Autodesk Inventor part; units mm, degrees
ref_plane "YZ Plane" through (0, 0, 0) normal (1, 0, 0) x (0, 1, 0)
ref_plane "XZ Plane" through (0, 0, 0) normal (0, 1, 0) x (-1, 0, 0)
ref_plane "XY Plane" through (0, 0, 0) normal (0, 0, 1) x (1, 0, 0)
sketch "Sketch1" plane through (0, 0, 0) normal (0, 0, 1) x (1, 0, 0)
  line L0 (0, 0) -> (-2.0828, 0)
  line L1 (-2.0828, 0) -> (-2.0828, 9.144)
  line L2 (-2.0828, 9.144) -> (0, 9.144)
  line L3 (0, 9.144) -> (0, 0)
  line L4 (-2.0828, 9.144) -> (-3.81, 11.176)
  line L5 (-3.81, 11.176) -> (-3.81, 11.684)
  line L6 (-3.81, 11.684) -> (0, 11.684)
  line L7 (0, 11.684) -> (0, 9.144)
  dimension "d0" = 4.1656
  dimension "d1" = 9.144
  dimension "d2" = 7.62
  dimension "d3" = 0.508
  dimension "d4" = 2.54
revolve "Revolution1" add sketch "Sketch1" angle 360 about axis through (0, 9.144, 0) along (0, -1, 0)
thread "Thread1"
sketch "Sketch2" plane through (0, 11.684, 0) normal (0, 1, 0) x (1, 0, 0)
  circle A0 centre (0, 0) radius 3.81
  line L0 (2.54, 0.635) -> (2.54, -0.635)
  line L1 (-2.54, -0.635) -> (-2.54, 0.635)
  line L2 (-0.635, 2.54) -> (0.635, 2.54)
  line L3 (0.635, -2.54) -> (-0.635, -2.54)
  line L4 (-0.635, -2.54) -> (-0.635, -1.397)
  line L5 (-0.635, 1.397) -> (-0.635, 2.54)
  line L6 (2.54, -0.635) -> (1.397, -0.635)
  line L7 (-1.397, -0.635) -> (-2.54, -0.635)
  line L8 (0.635, 2.54) -> (0.635, 1.397)
  line L9 (0.635, -1.397) -> (0.635, -2.54)
  line L10 (-2.54, 0.635) -> (-1.397, 0.635)
  line L11 (1.397, 0.635) -> (2.54, 0.635)
  line L12 (0, 2.54) -> (0, 0) construction
  line L13 (0, 0) -> (-2.54, 0) construction
  arc A1 (-0.635, -1.397) -> (-1.397, -0.635) centre (-1.397, -1.397) ccw
  arc A2 (1.397, -0.635) -> (0.635, -1.397) centre (1.397, -1.397) ccw
  arc A3 (0.635, 1.397) -> (1.397, 0.635) centre (1.397, 1.397) ccw
  arc A4 (-1.397, 0.635) -> (-0.635, 1.397) centre (-1.397, 1.397) ccw
  dimension "d8" = 1.27
  dimension "d9" = 5.08
  dimension "d10" = 0.762
extrude "Extrusion1" cut sketch "Sketch2" against normal blind 2.54 draft -14 contours L0 L6 A2 L9 L3 L4 A1 L7 L1 L10 A4 L5 L2 L8 A3 L11
chamfer "Chamfer1" distance 0.254 angle 45 1 edges at (2.0828, 0, 0)
properties material "Steel"
Geometry: final body of the model. Coordinates: model frame, mm. A direction names the side the tool comes from. Round coordinates to 2 decimals unless told otherwise and drop trailing zeros. Loops run counter-clockwise (first coordinate to the right, second up) from the corner with the lowest first, then second, coordinate; pieces in that order, holes last.
Item 1: Contact query for flat-ended pins moving along their axis: P1, Ø3, axis at x = 2.5, y = 6, coming from the -Z side; P2, Ø1.5, axis at y = 4, z = -1.5, coming from the +X side; P3, Ø3, axis at y = 6, z = -1, coming from the -X side. Output: stop coordinate, or through.
Checked values:
P1: stops at z = -1.83
P2: stops at x = 1.94
P3: stops at x = -2.08
Item 2: Section A-A, the plane y = 6.75. Output: boundary loops of the cut face in (x, z), plus the area to 3 significant figures.
Checked values:
outline: circle Ø4.17 at (0, 0)
area: 13.6 mm2
Item 3: Line query: L1, parallel to Z at x = 1, y = 8.5; L2, parallel to Z at x = 2, y = 10.5. Output: solid intervals per line, ascending.
Checked values:
L1: z = -1.83 to 1.83
L2: z = -2.54 to -0.34, 0.34 to 2.54
Item 4: Reachability of faces 1 (the flat face through (0, 0, 0)), 2 (the cylindrical face through (-1.987, 4.761, 0.626)), 3 (the flat face through (0.009, 10.714, 2.298)) from +Z, -Z, +X, -X, +Y, -Y: full face, straight path, thin tool, end or side. Return the list, or none.
Checked values:
face 1: +Z, -Z, +X, -X, -Y
face 2: -Y
face 3: +Y
Item 5: Mould query, pull axis Z, two halves, no side actions, for faces 4 (the flat face through (0.393, 10.714, -1.85)), 5 (the cylindrical face through (0.83, 11.43, -3.72)), 6 (the flat face through (1, 11.684, -1)), 7 (the flat face through (1.833, 10.714, -0.393)). Classes: released by +Z, released by -Z, zero draft, split by the parting line, or undercut.
Checked values:
face 4: undercut
face 5: split by the parting line
face 6: zero draft
face 7: undercut
